The listing builds one solid part. Answer for the finished solid, in the listing's coordinates (mm). Face numbers are marked on the shaded views. A direction names the side the tool comes from. Coordinates: 2 decimals unless noted, no trailing zeros. Order: outer loops, then holes, each group sorted by start corner. A loop starts at its lowest first (then second) coordinate and runs counter-clockwise, first axis right, second up. Notation, with made-up numbers: (60, 45.25) -> (80, 45.25) arc R5 cw to (80, 52.25) -> close; hole circle Ø6 at (41, 27.5). An arc over 180 degrees is marked (long way). Answer in a Markdown table with one row per item.
```python
from build123d import *

# Parameters (mm, degrees)
F1_DEPTH = 23.622
F2_R     = 5.08


with BuildPart() as f1:
    # F0 (on Top) → F1 (new body)
    with BuildSketch(Plane.XY):
        with BuildLine():
            Line((16.000509, 14.004066), (16.000509, 22.72998))
            ThreePointArc((16.000509, 22.72998), (7.887729, 58.203177), (1.843651, 22.31956))
            Line((1.843651, 22.31956), (1.843651, -45.733988))
            Line((1.843651, -45.733988), (1.762765, -49.65125))
            Line((1.762765, -49.65125), (16.000544, -49.65125))
            Line((16.000544, -49.65125), (16.000544, -29.869115))
            Line((16.000544, -29.869115), (40.347772, -29.869094))
            Line((40.347772, -29.869094), (40.347763, -19.096614))
            Line((40.347763, -19.096614), (16.000538, -19.096635))
            Line((16.000538, -19.096635), (16.000544, -6.953149))
            Line((16.000544, -6.953149), (34.080159, -6.953133))
            Line((34.080159, -6.953133), (34.080148, 5.973834))
            Line((34.080148, 5.973834), (16.000516, 5.973818))
            Line((16.000516, 5.973818), (16.000509, 14.004066))
        make_face()
    extrude(amount=F1_DEPTH)

    # F2
    f2_edges = [f1.edges().sort_by_distance(p)[0] for p in [
        (40.347768, -24.482854, 23.622),
        (34.080154, -0.48965, 23.622),
        (8.881655, -49.65125, 23.622),
        (34.080154, -0.48965, 0),
        (40.347768, -24.482854, 0),
        (8.881655, -49.65125, 0),
    ]]
    fillet(f2_edges, radius=F2_R)


solid = f1.part
```
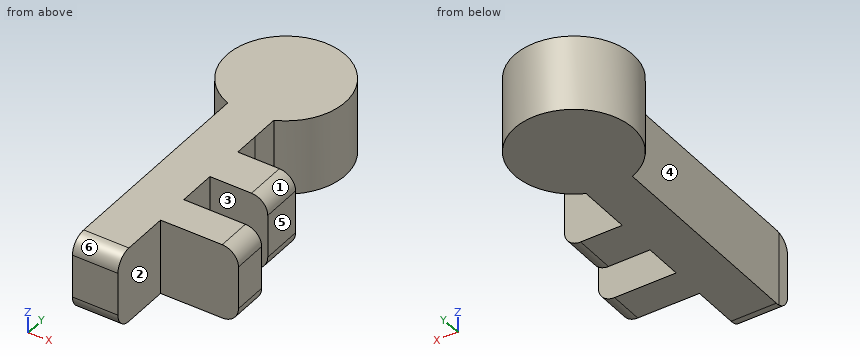
(1) Which of the six approach directions +Z, -Z, +X, -X, +Y, -Y give full straight-line access (tool end or side, diameter ignored) to the marked faces 1, 2 and 3?
Check values:
| item | result |
|---|---|
| face 1 | +Z, +X, +Y |
| face 2 | +Z, -Z, +X, -Y |
| face 3 | +Z, -Z, +X |
(2) Find the intervals of material crossed by line 1 along Y through (x, z) = (27.5, 6.5); line 2 along Y through (x, z) = (23.5, 8.75); line 3 along Y through (x, z) = (19.5, 20), in increasing order. Write a range as from..to.
Check values:
| item | result |
|---|---|
| line 1 | -29.87..-19.1, -6.95..5.97 |
| line 2 | -29.87..-19.1, -6.95..5.97, 28.85..50.47 |
| line 3 | -29.87..-19.1, -6.95..5.97, 24.78..54.54 |
(3) A cutting plane is placed at B-B, the plane x = 19. Determine the outline of the cut face in (y, z).
Check values:
| item | result |
|---|---|
| outline | (-29.87, 0) -> (-19.1, 0) -> (-19.1, 23.62) -> (-29.87, 23.62) -> close; (-6.95, 0) -> (5.97, 0) -> (5.97, 23.62) -> (-6.95, 23.62) -> close; (24.42, 0) -> (54.9, 0) -> (54.9, 23.62) -> (24.42, 23.62) -> close |
(4) A cutting plane is placed at D-D, the plane y = -15.5. Determine the outline of the cut face in (x, z).
Check values:
| item | result |
|---|---|
| outline | (1.84, 0) -> (16, 0) -> (16, 23.62) -> (1.84, 23.62) -> close |
(5) Flat-ended cylindrical pins translate along their axes: pin 1 (10.5 mm diameter, centred on y = 1.5, z = 11, fed in from +X); pin 2 (9 mm diameter, centred on x = 21.5, z = 7.5, fed in from +Y); pin 3 (10 mm diameter, centred on x = -2.5, z = 13, fed in from +Y); pin 4 (1 mm diameter, centred on x = 29.5, y = 3, fed in from -Z). Find the tip coordinate at first contact, or state that the pin passes through.
Check values:
| item | result |
|---|---|
| pin 1 | x = 34.08 |
| pin 2 | y = 56.11 |
| pin 3 | y = 57.24 |
| pin 4 | z = 0 |
(6) A cutting plane is placed at C-C, the plane x = 28. Determine the outline of the cut face in (y, z), then the cut area to 3 significant figures.
Check values:
| item | result |
|---|---|
| outline | (-29.87, 0) -> (-19.1, 0) -> (-19.1, 23.62) -> (-29.87, 23.62) -> close; (-6.95, 0) -> (5.97, 0) -> (5.97, 23.62) -> (-6.95, 23.62) -> close |
| area | 560 mm² |
(7) For a pull along Y with two mould halves and no side action, classify the marked faces 4, 5 and 6 as released by +Y, released by -Y, zero draft, split by the parting line, or undercut.
Check values:
| item | result |
|---|---|
| face 4 | undercut |
| face 5 | zero draft |
| face 6 | released by -Y |
(8) A cutting plane is placed at A-A, the plane z = 8.75. Determine the outline of the cut face in (x, y), then the cut area to 3 significant figures.
Check values:
| item | result |
|---|---|
| outline | (1.76, -49.65) -> (16, -49.65) -> (16, -29.87) -> (40.35, -29.87) -> (40.35, -19.1) -> (16, -19.1) -> (16, -6.95) -> (34.08, -6.95) -> (34.08, 5.97) -> (16, 5.97) -> (16, 14) -> (16, 22.73) arc R18.55 ccw (long way) to (1.84, 22.32) -> (1.84, -45.73) -> close |
| area | 2,590 mm² |
